Work out the finished part from the listing and answer in its coordinate system (mm). A direction names the side the tool comes from. Give positions to 0.01 mm unless a question says otherwise; leave off trailing zeros. Order: outer loops, then holes, each group sorted by start corner. A loop starts at its lowest first (then second) coordinate and runs counter-clockwise, first axis right, second up. Notation, with made-up numbers: (55.25, 88) - (114.25, 88) arc R24 ccw to (114.25, 127) - close; hole circle Ø10 at (43.5, 11.25). An arc over 180 degrees is marked (long way). Put each result on its own line as item: value.
Solid Edge part; units mm, degrees
sketch "Sketch1" plane through (0, 0, 0) normal (0, 0, 1) x (1, 0, 0)
  line L0 (70, 10) -> (0, 10)
  line L1 (0, 10) -> (0, 0)
  line L2 (0, 0) -> (70, 0)
  line L3 (70, 0) -> (70, 10)
extrude "Protrusion1" add sketch "Sketch1" along normal blind 90
hole "Hole_1" at (7, 0, 54) direction (0, 1, 0) diameter 4.134 end up to next start chamfer 0.6 start chamfer angle 45 end chamfer 0.6 end chamfer angle 45 thread major 5 thread length 2
hole "Hole1" at (67, 0, 54) direction (0, 1, 0) diameter 4.134 end up to next start chamfer 0.6 start chamfer angle 45 end chamfer 0.6 end chamfer angle 45 thread major 5 thread length 2
hole "Hole2" at (67, 0, 84) direction (0, 1, 0) diameter 4.134 end up to next start chamfer 0.6 start chamfer angle 45 end chamfer 0.6 end chamfer angle 45 thread major 5 thread length 2
hole "Hole3" at (7, 0, 84) direction (0, 1, 0) diameter 4.134 end up to next start chamfer 0.6 start chamfer angle 45 end chamfer 0.6 end chamfer angle 45 thread major 5 thread length 2
hole "Hole_5" at (10, 5, 0) direction (0, 0, 1) diameter 3.242 depth 30 start chamfer 0.6 start chamfer angle 45 thread major 4 thread length 2
hole "Hole4" at (40, 5, 0) direction (0, 0, 1) diameter 3.242 depth 30 start chamfer 0.6 start chamfer angle 45 thread major 4 thread length 2
(1) Section D-D, the plane x = 40 is taken. Write down the section's boundary in (y, z).
Geometry check:
outline: (0, 0) - (2.78, 0) - (3.38, 0.6) - (3.38, 30) - (6.62, 30) - (6.62, 0.6) - (7.22, 0) - (10, 0) - (10, 90) - (0, 90) - close
(2) Given pin 1 (1 mm diameter, centred on x = 9.5, y = 5, fed in from -Z), flat-ended and moving along its own axis, determine where the tip first touches the part or whether it passes through.
Geometry check:
pin 1: stops at z = 30
(3) Section B-B, the plane z = 54 is taken. Write down the section's boundary in (x, y), then the cut area to 3 significant figures.
Geometry check:
outline: (0, 0) - (4.33, 0) - (4.93, 0.6) - (4.93, 9.4) - (4.33, 10) - (0, 10) - close; (9.07, 0.6) - (9.67, 0) - (64.33, 0) - (64.93, 0.6) - (64.93, 9.4) - (64.33, 10) - (9.67, 10) - (9.07, 9.4) - close; (69.07, 0.6) - (69.67, 0) - (70, 0) - (70, 10) - (69.67, 10) - (69.07, 9.4) - close
area: 616 mm²
(4) Section A-A, the plane x = 67 is taken. Write down the section's boundary in (y, z).
Geometry check:
outline: (0, 0) - (10, 0) - (10, 51.33) - (9.4, 51.93) - (0.6, 51.93) - (0, 51.33) - close; (0, 56.67) - (0.6, 56.07) - (9.4, 56.07) - (10, 56.67) - (10, 81.33) - (9.4, 81.93) - (0.6, 81.93) - (0, 81.33) - close; (0, 86.67) - (0.6, 86.07) - (9.4, 86.07) - (10, 86.67) - (10, 90) - (0, 90) - close
(5) Straight lines are drawn through the part: line 1 (X direction, y = 5, z = 18.75); line 2 (X direction, y = 5.25, z = 54); line 3 (Z direction, x = 6, y = 3.5). For each, find the intervals that lie inside material, in ascending order.
Geometry check:
line 1: x = 0 to 8.38, 11.62 to 38.38, 41.62 to 70
line 2: x = 0 to 4.93, 9.07 to 64.93, 69.07 to 70
line 3: z = 0 to 52.19, 55.81 to 82.19, 85.81 to 90
(6) Determine the mould class of faces 3 (the face through (35, 10, 44)), 4 (the face through (7.091, 4.938, 56.065)), 5 (the face through (70, 5, 44)), 6 (the face through (65.74, 4.94, 85.64)) for opening direction X: pulls with the +X half, pulls with the -X half, needs draft (parallel to the pull), parting line crosses it, or undercut.
Geometry check:
face 3: needs draft
face 4: undercut
face 5: pulls with the +X half
face 6: undercut
(7) Section C-C, the plane y = 5 is taken. Write down the section's boundary in (x, z).
Geometry check:
outline: (0, 0) - (7.78, 0) - (8.38, 0.6) - (8.38, 30) - (11.62, 30) - (11.62, 0.6) - (12.22, 0) - (37.78, 0) - (38.38, 0.6) - (38.38, 30) - (41.62, 30) - (41.62, 0.6) - (42.22, 0) - (70, 0) - (70, 90) - (0, 90) - close; hole circle Ø4.13 at (7, 54); hole circle Ø4.13 at (7, 84); hole circle Ø4.13 at (67, 54); hole circle Ø4.13 at (67, 84)
(8) A tool of negligible diameter and unlimited length cuts with its end or side. For faces 1 (the face through (40, 5, 30)), 2 (the face through (35, 5, 90)), from which of +Z, -Z, +X, -X, +Y, -Y can it reach the whole face along a straight path? Write none if from no direction.
Geometry check:
face 1: -Z
face 2: +Z, +X, -X, +Y, -Y
